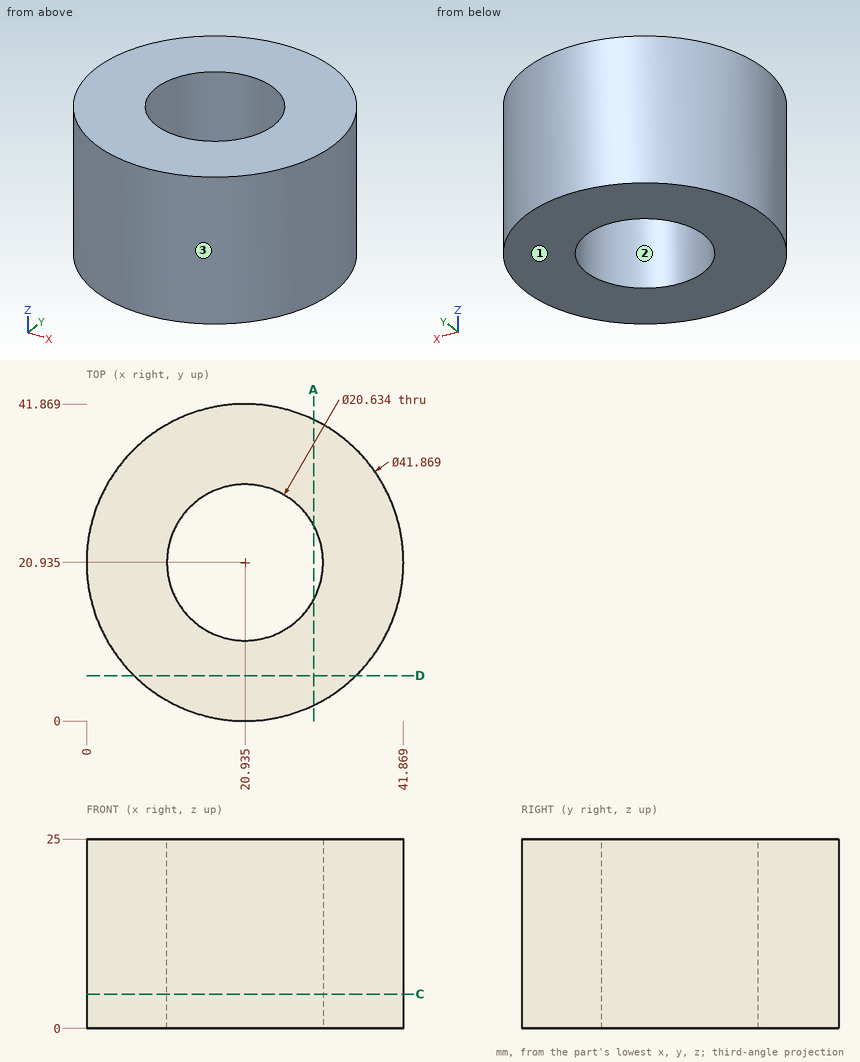
Study the drawing (mm; zero at the part's minimum x, y, z) and answer. Give positions to 0.01 mm unless a question says otherwise; leave off trailing zeros. Loops run counter-clockwise (first coordinate to the right, second up) from the corner with the lowest first, then second, coordinate; pieces in that order, holes last. Notation, with made-up numbers: (-23, -8) - (9, -8) arc R17 cw to (9, 17) - close; hole circle Ø8 at (-13, -28.75). An arc over 180 degrees is marked (long way). Return JSON: item names as keys, results as strings. Group by question number.
1. Given pin 1 Ø8 at (y, z) = (4, 19.5) entering from +X (1 decimal); pin 2 Ø5 at (x, z) = (17, 4) entering from +Y; pin 3 Ø3 at (x, y) = (14, 25.5) entering from -Z; pin 4 Ø4 at (x, z) = (32.5, 15.5) entering from +Y, each flat-ended and moving along its own axis, determine where each tip first touches the part or whether it passes through.
2. Determine the mould class of the marked faces 1, 2 and 3 for opening direction Y: pulls with the +Y half, pulls with the -Y half, needs draft (parallel to the pull), parting line crosses it, or undercut.
3. Find section C-C (z = 4.5). Write down the section's boundary in (x, y) (1 decimal), then the cut area to 3 significant figures.
4. Straight lines are drawn through the part: line 1 (X direction, y = 20, z = 9.75); line 2 (Y direction, x = 18, z = 21.25) (1 decimal); line 3 (Y direction, x = 25.5, z = 18) (1 decimal). For each, find the intervals that lie inside material, in ascending order. Write a range as [from, to].
5. Find section A-A (x = 30). Write down the section's boundary in (y, z) (1 decimal), then the cut area to 3 significant figures.
6. Find section D-D (y = 6). Write down the section's boundary in (x, z) (1 decimal).
Verdict:
{
 "1": {"pin 1": "stops at x = 37.4", "pin 2": "stops at y = 41.82", "pin 3": "passes through", "pin 4": "stops at y = 39.56"},
 "2": {"face 1": "needs draft", "face 2": "undercut", "face 3": "parting line crosses it"},
 "3": {"outline": "circle Ø41.9 at (20.9, 20.9); hole circle Ø20.6 at (20.9, 20.9)", "area": "1,040 mm^2"},
 "4": {"line 1": "x = [0.02, 10.66], [31.21, 41.85]", "line 2": "y = [0.2, 11], [30.8, 41.7]", "line 3": "y = [0.5, 11.7], [30.2, 41.4]"},
 "5": {"outline": "(2.1, 0) - (16, 0) - (16, 25) - (2.1, 25) - close; (25.9, 0) - (39.8, 0) - (39.8, 25) - (25.9, 25) - close", "area": "697 mm^2"},
 "6": {"outline": "(6.3, 0) - (35.6, 0) - (35.6, 25) - (6.3, 25) - close"}
}
